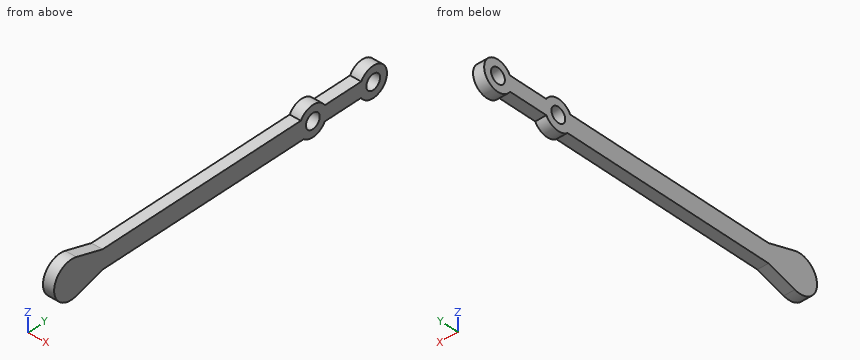
```python
from build123d import *

# Parameters (mm, degrees)
ESQUISSE1_W         = 3
ESQUISSE1_H         = 5
BOSS_EXTRU_1_DEPTH  = 65
BOSS_EXTRUDE1_START = -3
BOSS_EXTRUDE1_DEPTH = 3
ESQUISSE3_R         = 2
BOSS_EXTRUDE3_DEPTH = 3
ESQUISSE3_10_R      = 2
CUT_EXTRUDE2_DEPTH  = 10


# Read off the part's stored shape, not the designer's step: Boss-Extrude1
with BuildPart() as part:
    # Esquisse1 → Boss.-Extru.1 (new body)
    with BuildSketch(Plane(origin=(0, 0, 0), x_dir=(1, 0, 0), z_dir=(0, 1, 0))):
        Rectangle(ESQUISSE1_W, ESQUISSE1_H)
    extrude(amount=BOSS_EXTRU_1_DEPTH)

    # Boss-Extrude1 outline → Boss-Extrude1 (add)
    with BuildSketch(Plane.ZY.offset(1.5).offset(BOSS_EXTRUDE1_START)):
        with BuildLine():
            Line((4.792700519, -3.558056958), (2.5, 4.054226947))
            Line((2.5, 4.054226947), (2.5, 0))
            Line((2.5, 0), (-2.5, 0))
            Line((-2.5, 0), (-2.5, 4.054226947))
            Line((-2.5, 4.054226947), (-4.784214598, -3.563976926))
            ThreePointArc((-4.784214598, -3.563976926), (0.008223214, -9.999996411), (4.792700519, -3.558056958))
        make_face()
    extrude(amount=BOSS_EXTRUDE1_DEPTH)

    # Esquisse3 → Boss-Extrude3 (add, through all)
    with BuildSketch(Plane.ZY.offset(1.5)):
        with BuildLine():
            ThreePointArc((2.5, 79.034286522), (0.5, 86.498388137), (-1.5, 79.034286522))
            Line((-1.5, 79.034286522), (-1.5, 68.462489753))
            ThreePointArc((-1.5, 68.462489753), (0.5, 60.998388137), (2.5, 68.462489753))
            Line((2.5, 68.462489753), (2.5, 79.034286522))
        make_face()
        with Locations((0.5, 82.498388137)):
            Circle(ESQUISSE3_R, mode=Mode.SUBTRACT)
        with Locations((0.5, 64.998388137)):
            Circle(ESQUISSE3_R, mode=Mode.SUBTRACT)
    extrude(amount=-BOSS_EXTRUDE3_DEPTH)

    # Esquisse3<10> → Cut-Extrude2 (cut)
    with BuildSketch(Plane.ZY.offset(1.5)):
        with Locations((0.5, 64.998388137)):
            Circle(ESQUISSE3_10_R)
    extrude(amount=-CUT_EXTRUDE2_DEPTH, mode=Mode.SUBTRACT)


solid = part.part
```
For this review, take the finished solid that the model builds, in its own axes (mm). Give positions to 0.01 mm unless a question says otherwise; leave off trailing zeros. Loops run counter-clockwise (first coordinate to the right, second up) from the corner with the lowest first, then second, coordinate; pieces in that order, holes last. Notation, with made-up numbers: M -15.75,-6.75 L 20.25,-6.75 A7 ccw 20.25,1.25 Z; hole C 64,70.5 d5. An arc over 180 degrees is marked long. One line per item, written item: value. Start each with the question number.
Q1. Add section D-D (y = 0.5). Give the boundary of the cut face in (x, z), and give its area (3 significant figures).
Q2. Clearance check with flat-ended pins moving along their axes: pin 1 Ø2.5 at (y, z) = (82.5, 0.5) entering from +X; pin 2 Ø0.9 at (x, y) = (-0.5, 72.5) entering from -Z; pin 3 Ø1.5 at (x, y) = (0.5, 74.5) entering from +Z. State where each tip first meets the part, or that it passes through.
Q3. Add section B-B (x = -0.3). Give the boundary of the cut face in (y, z), and give its area (3 significant figures).
Q4. Add section C-C (y = 40.5). Give the boundary of the cut face in (x, z).
Q5. For L1, parallel to Y at x = 1.4, z = 0.25; L2, parallel to Y at x = 1.3, z = -1.25; L3, parallel to Z at x = -1, y = 34, list the stretches that pass through material, from the lowest coordinate up.
Q6. Add section A-A (z = 0.5). Give the boundary of the cut face in (x, y).
Reply:
1. outline: M -1.5,-3.57 L 1.5,-3.57 L 1.5,3.57 L -1.5,3.57 Z
1. area: 21.4 mm²
2. pin 1: through
2. pin 2: z = -1.5
2. pin 3: z = 2.5
3. outline: M -3.56,-4.78 L 4.05,-2.5 L 62.35,-2.5 A4 ccw 68.46,-1.5 L 79.03,-1.5 A4 ccw long 79.03,2.5 L 68.46,2.5 A4 ccw 61.53,2.5 L 4.05,2.5 L -3.56,4.79 A5 ccw long Z; hole C 65,0.5 d4; hole C 82.5,0.5 d4
3. area: 510 mm²
4. outline: M -1.5,-2.5 L 1.5,-2.5 L 1.5,2.5 L -1.5,2.5 Z
5. L1: -9.99 to 63.01, 66.98 to 80.51, 84.48 to 86.49
5. L2: -9.84 to 64.03, 65.97 to 81.53, 83.47 to 86.1
5. L3: -2.5 to 2.5
6. outline: M -1.5,-9.98 L 1.5,-9.98 L 1.5,63 L -1.5,63 Z; M -1.5,67 L 1.5,67 L 1.5,80.5 L -1.5,80.5 Z; M -1.5,84.5 L 1.5,84.5 L 1.5,86.5 L -1.5,86.5 Z
